```python
from build123d import *

# Parameters (mm, degrees)
SKETCH1_R           = 7
SKETCH1_R_2         = 3
BOSS_EXTRUDE1_DEPTH = 20
SKETCH2_R           = 10
SKETCH2_R_2         = 3
BOSS_EXTRUDE2_DEPTH = 20
CUT_EXTRUDE2_DEPTH  = 20
SKETCH4_R           = 21.655225415
SKETCH4_R_2         = 6
CUT_EXTRUDE3_DEPTH  = 20
SKETCH6_R           = 3.1
CUT_EXTRUDE4_DEPTH  = 80


with BuildPart() as part:
    # Sketch1 → Boss-Extrude1 (new body)
    with BuildSketch(Plane(origin=(0, 0, 0), x_dir=(1, 0, 0), z_dir=(0, 1, 0))):
        with Locations(Location((0, 0, 0), (0, 0, 270))):  # turned: the seam where the file's is
            Circle(SKETCH1_R)
        with Locations(Location((0, 0, 0), (0, 0, 270))):  # turned: the seam where the file's is
            Circle(SKETCH1_R_2, mode=Mode.SUBTRACT)
    extrude(amount=BOSS_EXTRUDE1_DEPTH)

    # Sketch2 → Boss-Extrude2 (add)
    with BuildSketch(Plane(origin=(0, 20, 0), x_dir=(1, 0, 0), z_dir=(0, 1, 0))):
        with Locations(Location((0, 0, 0), (0, 0, 270))):  # turned: the seam where the file's is
            Circle(SKETCH2_R)
        with Locations(Location((0, 0, 0), (0, 0, 270))):  # turned: the seam where the file's is
            Circle(SKETCH2_R_2, mode=Mode.SUBTRACT)
    extrude(amount=BOSS_EXTRUDE2_DEPTH)

    # Sketch3 → Cut-Extrude2 (cut)
    with BuildSketch(Plane(origin=(0, 40, 0), x_dir=(1, 0, 0), z_dir=(0, 1, 0))):
        with BuildLine():
            Line((1.481181144, 7.809519004), (3.294093052, 9.441872217))
            ThreePointArc((3.294093052, 9.441872217), (1.777835424, 9.840696175), (0.217876864, 9.997626202))
            Line((0.217876864, 9.997626202), (1.481181144, 7.809519004))
        make_face()
        with BuildLine():
            ThreePointArc((6.050567636, 7.961823364), (4.731764319, 8.809676863), (3.296649611, 9.440979893))
            Line((3.296649611, 9.440979893), (3.821961069, 6.969583792))
            Line((3.821961069, 6.969583792), (6.050567636, 7.961823364))
        make_face()
        with BuildLine():
            Line((-1.004587111, 7.885004083), (0.215169688, 9.997684832))
            ThreePointArc((0.215169688, 9.997684832), (-1.35012039, 9.908439581), (-2.882223189, 9.5756352))
            Line((-2.882223189, 9.5756352), (-1.004587111, 7.885004083))
        make_face()
        with BuildLine():
            ThreePointArc((8.214770503, 5.702415767), (7.222515155, 6.916304999), (6.052723325, 7.960184693))
            Line((6.052723325, 7.960184693), (5.788620815, 5.447417159))
            Line((5.788620815, 5.447417159), (8.214770503, 5.702415767))
        make_face()
        with BuildLine():
            Line((-3.392019381, 7.188650024), (-2.884815983, 9.574854398))
            ThreePointArc((-2.884815983, 9.574854398), (-4.345917013, 9.006275885), (-5.700191154, 8.216314308))
            Line((-5.700191154, 8.216314308), (-3.392019381, 7.188650024))
        make_face()
        with BuildLine():
            ThreePointArc((9.574854398, 2.884815983), (9.006275885, 4.345917013), (8.216314308, 5.700191154))
            Line((8.216314308, 5.700191154), (7.188650024, 3.392019381))
            Line((7.188650024, 3.392019381), (9.574854398, 2.884815983))
        make_face()
        with BuildLine():
            Line((-5.447417159, 5.788620815), (-5.702415767, 8.214770503))
            ThreePointArc((-5.702415767, 8.214770503), (-6.916304999, 7.222515155), (-7.960184693, 6.052723325))
            Line((-7.960184693, 6.052723325), (-5.447417159, 5.788620815))
        make_face()
        with BuildLine():
            ThreePointArc((9.997684832, -0.215169688), (9.908439581, 1.35012039), (9.5756352, 2.882223189))
            Line((9.5756352, 2.882223189), (7.885004083, 1.004587111))
            Line((7.885004083, 1.004587111), (9.997684832, -0.215169688))
        make_face()
        with BuildLine():
            Line((-6.969583792, 3.821961069), (-7.961823364, 6.050567636))
            ThreePointArc((-7.961823364, 6.050567636), (-8.809676863, 4.731764319), (-9.440979893, 3.296649611))
            Line((-9.440979893, 3.296649611), (-6.969583792, 3.821961069))
        make_face()
        with BuildLine():
            ThreePointArc((9.441872217, -3.294093052), (9.840696175, -1.777835424), (9.997626202, -0.217876864))
            Line((9.997626202, -0.217876864), (7.809519004, -1.481181144))
            Line((7.809519004, -1.481181144), (9.441872217, -3.294093052))
        make_face()
        with BuildLine():
            Line((-7.809519004, 1.481181144), (-9.441872217, 3.294093052))
            ThreePointArc((-9.441872217, 3.294093052), (-9.840696175, 1.777835424), (-9.997626202, 0.217876864))
            Line((-9.997626202, 0.217876864), (-7.809519004, 1.481181144))
        make_face()
        with BuildLine():
            ThreePointArc((7.961823364, -6.050567636), (8.809676863, -4.731764319), (9.440979893, -3.296649611))
            Line((9.440979893, -3.296649611), (6.969583792, -3.821961069))
            Line((6.969583792, -3.821961069), (7.961823364, -6.050567636))
        make_face()
        with BuildLine():
            Line((-7.885004083, -1.004587111), (-9.997684832, 0.215169688))
            ThreePointArc((-9.997684832, 0.215169688), (-9.908439581, -1.35012039), (-9.5756352, -2.882223189))
            Line((-9.5756352, -2.882223189), (-7.885004083, -1.004587111))
        make_face()
        with BuildLine():
            ThreePointArc((5.702415767, -8.214770503), (6.916304999, -7.222515155), (7.960184693, -6.052723325))
            Line((7.960184693, -6.052723325), (5.447417159, -5.788620815))
            Line((5.447417159, -5.788620815), (5.702415767, -8.214770503))
        make_face()
        with BuildLine():
            Line((-7.188650024, -3.392019381), (-9.574854398, -2.884815983))
            ThreePointArc((-9.574854398, -2.884815983), (-9.006275885, -4.345917013), (-8.216314308, -5.700191154))
            Line((-8.216314308, -5.700191154), (-7.188650024, -3.392019381))
        make_face()
        with BuildLine():
            ThreePointArc((2.884815983, -9.574854398), (4.345917013, -9.006275885), (5.700191154, -8.216314308))
            Line((5.700191154, -8.216314308), (3.392019381, -7.188650024))
            Line((3.392019381, -7.188650024), (2.884815983, -9.574854398))
        make_face()
        with BuildLine():
            Line((-5.788620815, -5.447417159), (-8.214770503, -5.702415767))
            ThreePointArc((-8.214770503, -5.702415767), (-7.222515155, -6.916304999), (-6.052723325, -7.960184693))
            Line((-6.052723325, -7.960184693), (-5.788620815, -5.447417159))
        make_face()
        with BuildLine():
            ThreePointArc((-0.215169688, -9.997684832), (1.35012039, -9.908439581), (2.882223189, -9.5756352))
            Line((2.882223189, -9.5756352), (1.004587111, -7.885004083))
            Line((1.004587111, -7.885004083), (-0.215169688, -9.997684832))
        make_face()
        with BuildLine():
            Line((-3.821961069, -6.969583792), (-6.050567636, -7.961823364))
            ThreePointArc((-6.050567636, -7.961823364), (-4.731764319, -8.809676863), (-3.296649611, -9.440979893))
            Line((-3.296649611, -9.440979893), (-3.821961069, -6.969583792))
        make_face()
        with BuildLine():
            ThreePointArc((-3.294093052, -9.441872217), (-1.777835424, -9.840696175), (-0.217876864, -9.997626202))
            Line((-0.217876864, -9.997626202), (-1.481181144, -7.809519004))
            Line((-1.481181144, -7.809519004), (-3.294093052, -9.441872217))
        make_face()
    extrude(amount=-CUT_EXTRUDE2_DEPTH, mode=Mode.SUBTRACT)

    # Sketch4 → Cut-Extrude3 (cut)
    with BuildSketch(Plane(origin=(0, 0, 0), x_dir=(-1, 0, 0), z_dir=(0, -1, 0))):
        with Locations((3.244661678, 1.192157737)):
            Circle(SKETCH4_R)
        with Locations(Location((0, 0, 0), (0, 0, 90))):  # turned: the seam where the file's is
            Circle(SKETCH4_R_2, mode=Mode.SUBTRACT)
    extrude(amount=-CUT_EXTRUDE3_DEPTH, mode=Mode.SUBTRACT)

    # Sketch6 → Cut-Extrude4 (cut)
    with BuildSketch(Plane(origin=(0, 0, 0), x_dir=(-1, 0, 0), z_dir=(0, -1, 0))):
        with Locations(Location((0, 0, 0), (0, 0, 90))):  # turned: the seam where the file's is
            Circle(SKETCH6_R)
    extrude(amount=-CUT_EXTRUDE4_DEPTH, mode=Mode.SUBTRACT)


solid = part.part
```
Geometry: final body of the model. Coordinates: model frame, mm. A direction names the side the tool comes from. Round coordinates to 2 decimals unless told otherwise and drop trailing zeros. Loops run counter-clockwise (first coordinate to the right, second up) from the corner with the lowest first, then second, coordinate; pieces in that order, holes last. Notation, with made-up numbers: (-12, -13.5) -> (6, -13.5) arc R13 ccw to (6, 9.5) -> close; hole circle Ø5 at (1, 60.5). An arc over 180 degrees is marked (long way). Use one line per item in the form item = value. Start each with the question number.
1) First-contact query: P1, Ø5, axis at y = 6, z = -1, coming from the +X side; P2, Ø3, axis at y = 35, z = -5, coming from the +X side; P3, Ø1.5, axis at y = 15.5, z = 3.5, coming from the +X side. Flat tips, straight axial feed; report the tip coordinate or a pass-through.
2) Draft query along Z for faces 1 (the flat face through (-5.573, 30.14, -6.985)), 2 (the flat face through (-3.14, 30.14, -8.37)), 3 (the flat face through (-3, 0, 3)), 4 (the flat face through (0.4, 30.14, 8.93)). Return one class per face: released by +Z, released by -Z, zero draft, split by the parting line, or undercut.
3) Section A-A on y = 17.5. Output: boundary loops of the cut face in (x, z), then the cut area to 3 significant figures.
4) Line query: L1, parallel to Z at x = 7.5, y = 28; L2, parallel to X at y = 11.5, z = 0; L3, parallel to Y at x = -7, z = -1.5. Output: solid intervals per line, ascending.
5) Access query for faces 5 (the flat face through (8.61, 30.14, 2.37)), 6 (the flat face through (-0.84, 30.14, 8.92)), 7 (the flat face through (5, 20, 4)), 8 (the flat face through (-4.56, 30.14, -7.71)). Directions: +Z, -Z, +X, -X, +Y, -Y. A direction counts if a zero-diameter tool reaches every point of the face in a straight line with its end or side. Return the directions, or none.
Response:
q1.P1 = 6
q1.P2 = 8.22
q1.P3 = 5.33
q2.face_1 = undercut
q2.face_2 = released by -Z
q2.face_3 = zero draft
q2.face_4 = released by +Z
q3.outline = circle Ø12 at (0, 0); hole circle Ø6.2 at (0, 0)
q3.area = 82.9 mm^2
q4.L1 = -5.63 to -4.09, -3.33 to 3.71, 5.01 to 6
q4.L2 = -6 to -3.1, 3.1 to 6
q4.L3 = 20 to 40
q5.face_5 = +X, +Y, -Y
q5.face_6 = +Z, +Y, -Y
q5.face_7 = -Y
q5.face_8 = -Z, +Y, -Y
